```python
from build123d import *

# Parameters (mm, degrees)
PAD004_DEPTH     = 11.7
SHAPEBINDER001_R = 4
PAD005_DEPTH     = 11.7
SKETCH008_R      = 1.5
POCKET004_DEPTH  = 7
FILLET002_R      = 5
SKETCH009_W      = 101
SKETCH009_H      = 76
POCKET005_DEPTH  = 6.7
SKETCH011_W      = 76
SKETCH011_H      = 38.25
SKETCH011_W_2    = 38
SKETCH011_H_2    = 19
POCKET006_DEPTH  = 3.5
SKETCH012_W      = 14
SKETCH012_H      = 14
POCKET007_DEPTH  = 1.5
SKETCH015_W      = 13
SKETCH015_H      = 7
POCKET010_DEPTH  = 5
SKETCH016_R      = 2.75
POCKET011_DEPTH  = 5
SKETCH017_W      = 5
SKETCH017_H      = 17
POCKET012_DEPTH  = 2.5
SKETCH018_W      = 3
SKETCH018_H      = 17
POCKET013_DEPTH  = 4.5
POCKET014_DEPTH  = 2
FILLET003_R      = 2


with BuildPart() as part:
    # ShapeBinder → Pad004 (new body)
    with BuildSketch(Plane(origin=(0, 0, 0), x_dir=(0, 1, 0), z_dir=(0, 0, 1))):
        with BuildLine():
            Line((43, -51.5), (43, 51.5))
            ThreePointArc((43, 51.5), (41.828427, 54.328427), (39, 55.5))
            Line((39, 55.5), (-39, 55.5))
            ThreePointArc((-39, 55.5), (-41.828427, 54.328427), (-43, 51.5))
            Line((-43, 51.5), (-43, -51.5))
            ThreePointArc((-43, -51.5), (-41.828427, -54.328427), (-39, -55.5))
            Line((-39, -55.5), (39, -55.5))
            ThreePointArc((39, -55.5), (41.828427, -54.328427), (43, -51.5))
        make_face()
    extrude(amount=PAD004_DEPTH)

    # ShapeBinder001 → Pad005 (join)
    with BuildSketch(Plane(origin=(0, 0, 0), x_dir=(0, 1, 0), z_dir=(0, 0, 1))):
        with Locations((42, -54.5)):
            Circle(SHAPEBINDER001_R)
        with Locations((42, 54.5)):
            Circle(SHAPEBINDER001_R)
        with Locations((-42, -54.5)):
            Circle(SHAPEBINDER001_R)
        with Locations((-42, 54.5)):
            Circle(SHAPEBINDER001_R)
    extrude(amount=PAD005_DEPTH)

    # Sketch008 (on Face8 of Pad005) → Pocket004 (cut)
    with BuildSketch(Plane.XY.offset(11.7)):
        with Locations((54.5, 42)):
            Circle(SKETCH008_R)
        with Locations((-54.5, 42)):
            Circle(SKETCH008_R)
        with Locations((-54.5, -42)):
            Circle(SKETCH008_R)
        with Locations((54.5, -42)):
            Circle(SKETCH008_R)
    extrude(amount=-POCKET004_DEPTH, mode=Mode.SUBTRACT)

    # Fillet002
    fillet002_edges = [part.edges().sort_by_distance(p)[0] for p in [
        (-55.5, -38.127017, 5.85),
        (-55.5, 38.127017, 5.85),
        (50.627017, 43, 5.85),
        (-50.627017, 43, 5.85),
        (55.5, -38.127017, 5.85),
        (55.5, 38.127017, 5.85),
        (-50.627017, -43, 5.85),
        (50.627017, -43, 5.85),
    ]]
    fillet(fillet002_edges, radius=FILLET002_R)

    # Sketch009 (on Face5 of Fillet002) → Pocket005 (cut)
    with BuildSketch(Plane.XY.offset(11.7)):
        Rectangle(SKETCH009_W, SKETCH009_H)
    extrude(amount=-POCKET005_DEPTH, mode=Mode.SUBTRACT)

    # Sketch011 (on Face30 of Pocket005) → Pocket006 (cut)
    with BuildSketch(Plane.XY.offset(5)):
        with Locations((-9.5, -15.125)):
            Rectangle(SKETCH011_W, SKETCH011_H)
        with Locations((28.5, 25.5)):
            Rectangle(SKETCH011_W_2, SKETCH011_H_2)
    extrude(amount=-POCKET006_DEPTH, mode=Mode.SUBTRACT)

    # Sketch012 (on Face40 of Pocket006) → Pocket007 (cut)
    with BuildSketch(Plane.XY.offset(1.5)):
        with Locations((-38, -5.5)):
            Rectangle(SKETCH012_W, SKETCH012_H)
        with Locations((-19, -5.5)):
            Rectangle(SKETCH012_W, SKETCH012_H)
        with Locations((0, -5.5)):
            Rectangle(SKETCH012_W, SKETCH012_H)
        with Locations((19, -5.5)):
            Rectangle(SKETCH012_W, SKETCH012_H)
        with Locations((-38, -24.75)):
            Rectangle(SKETCH012_W, SKETCH012_H)
        with Locations((-19, -24.75)):
            Rectangle(SKETCH012_W, SKETCH012_H)
        with Locations((0, -24.75)):
            Rectangle(SKETCH012_W, SKETCH012_H)
        with Locations((19, -24.75)):
            Rectangle(SKETCH012_W, SKETCH012_H)
        with Locations((19, 25.5)):
            Rectangle(SKETCH012_W, SKETCH012_H)
        with Locations((38, 25.5)):
            Rectangle(SKETCH012_W, SKETCH012_H)
    extrude(amount=-POCKET007_DEPTH, mode=Mode.SUBTRACT)

    # Sketch015 → Pocket010 (cut)
    with BuildSketch(Plane.XY.offset(5)):
        with Locations((44, -12)):
            Rectangle(SKETCH015_W, SKETCH015_H)
    extrude(amount=-POCKET010_DEPTH, mode=Mode.SUBTRACT)

    # Sketch016 (on Face1 of Pocket010) → Pocket011 (cut)
    with BuildSketch(Plane.YZ.offset(55.5)):
        with Locations((-12, 3)):
            Circle(SKETCH016_R)
    extrude(amount=-POCKET011_DEPTH, mode=Mode.SUBTRACT)

    # Sketch017 (on Face5 of Pocket007) → Pocket012 (cut)
    with BuildSketch(Plane.XY.offset(11.7)):
        with Locations((-53, 21.5)):
            Rectangle(SKETCH017_W, SKETCH017_H)
    extrude(amount=-POCKET012_DEPTH, mode=Mode.SUBTRACT)

    # Sketch018 (on Face73 of Pocket012) → Pocket013 (cut)
    with BuildSketch(Plane.XY.offset(9.2)):
        with Locations((-54, 21.5)):
            Rectangle(SKETCH018_W, SKETCH018_H)
    extrude(amount=-POCKET013_DEPTH, mode=Mode.SUBTRACT)

    # Sketch019 (on Face80 of Pocket013) → Pocket014 (cut)
    with BuildSketch(Plane(origin=(-52.5, 0, 0), x_dir=(0, -1, 0), z_dir=(-1, 0, 0))):
        with BuildLine():
            ThreePointArc((-25, 11.2), (-27, 9.2), (-25, 7.2))
            Line((-25, 7.2), (-18, 7.2))
            ThreePointArc((-18, 7.2), (-16, 9.2), (-18, 11.2))
            Line((-25, 11.2), (-18, 11.2))
        make_face()
    extrude(amount=-POCKET014_DEPTH, mode=Mode.SUBTRACT)

    # Fillet003
    fillet003_edges = [part.edges().sort_by_distance(p)[0] for p in [
        (-55.5, 21.5, 4.7),
        (-55.5, 30, 8.2),
        (-55.5, 13, 8.2),
    ]]
    fillet(fillet003_edges, radius=FILLET003_R)


solid = part.part
```
Design review of the part built by this model. Coordinates are the model's own, in mm. A direction names the side the tool comes from. Coordinates: 2 decimals unless noted, no trailing zeros. Loops run counter-clockwise (first coordinate to the right, second up) from the corner with the lowest first, then second, coordinate; pieces in that order, holes last.
Q1. We need section B-B on x = -14. State the section outline as (y, z) points, and give its area (3 significant figures).
Reported:
outline: (-43, 0) - (-31.75, 0) - (-31.75, 1.5) - (-34.25, 1.5) - (-34.25, 5) - (-38, 5) - (-38, 11.7) - (-43, 11.7) - close; (-17.75, 0) - (-12.5, 0) - (-12.5, 1.5) - (-17.75, 1.5) - close; (1.5, 0) - (43, 0) - (43, 11.7) - (38, 11.7) - (38, 5) - (4, 5) - (4, 1.5) - (1.5, 1.5) - close
area: 321 mm2
Q2. To check wall thickness, follow line 1 (Y direction, x = 54.5, z = 9.75); line 2 (Y direction, x = -44.5, z = 6); line 3 (X direction, y = 10, z = 8.75). State the ranges of each line that lie inside material, in increasing order.
Reported:
line 1: y = -46 to -43.5, -40.5 to 40.5, 43.5 to 46
line 2: y = -43 to -38, 38 to 43
line 3: x = -55.5 to -50.5, 50.5 to 55.5
Q3. For pin 1 (3 mm diameter, centred on x = -23.5, z = 9.5, fed in from -Y); pin 2 (1.2 mm diameter, centred on y = -4.5, z = 1, fed in from -X); pin 3 (5 mm diameter, centred on x = 54.5, y = -42, fed in from +Z); pin 4 (0.6 mm diameter, centred on x = -51, y = 15, fed in from +Z), all flat-tipped, find the tip position at first contact; note any pin that passes through.
Reported:
pin 1: stops at y = -43
pin 2: stops at x = -55.5
pin 3: stops at z = 11.7
pin 4: stops at z = 9.2
Q4. Tool access review of faces 5 (the face through (-1, 38, 8)), 6 (the face through (44, -15.5, 3)), 7 (the face through (55.948, 37.36, 5.768)), 8 (the face through (-55.924, -37.306, 5.768)): name each direction out of +Z, -Z, +X, -X, +Y, -Y from which nothing blocks a thin tool from reaching the whole face with its end or side.
Reported:
face 5: +Z
face 6: +Z, -Z
face 7: +Z, -Z, +X
face 8: +Z, -Z, -X
Q5. The part is to be moulded in two halves that separate along Y. For faces 1 (the face through (1, 43, 6)), 2 (the face through (44, -8.5, 3)), 3 (the face through (-1, 10, 0)), 4 (the face through (-49.86, -43.448, 5.768)), say which applies: +Y half, -Y half, draft (parallel to the pull), parting line (faces both ways), or undercut.
Reported:
face 1: +Y half
face 2: undercut
face 3: draft
face 4: -Y half
Q6. We need section A-A on x = 42.5. State the section outline as (y, z) points, and give its area (4 significant figures).
Reported:
outline: (-43, 0) - (-15.5, 0) - (-15.5, 5) - (-38, 5) - (-38, 11.7) - (-43, 11.7) - close; (-8.5, 0) - (18.5, 0) - (18.5, 1.5) - (16, 1.5) - (16, 5) - (-8.5, 5) - close; (32.5, 0) - (43, 0) - (43, 11.7) - (38, 11.7) - (38, 5) - (35, 5) - (35, 1.5) - (32.5, 1.5) - close
area: 374.5 mm2
